```python
from build123d import *

# Parameters (mm, degrees)
SKETCH12_W           = 12.7
SKETCH12_H           = 41.275
SKETCH12_R           = 2.5527
BOSS_EXTRUDE5_DEPTH  = 12.7
SKETCH13_R           = 2.0193
CUT_EXTRUDE3_DEPTH   = 13.7
SKETCH107_W          = 9.525
SKETCH107_H          = 11.1125
SKETCH107_R          = 2.0193
BOSS_EXTRUDE34_DEPTH = 12.7
SKETCH112_R          = 1.651
CUT_EXTRUDE58_DEPTH  = 13.7
FILLET43_R           = 2.54
FILLET44_R           = 0.635


with BuildPart() as part:
    # Sketch12 → Boss-Extrude5 (new body)
    with BuildSketch(Plane(origin=(0, 19.05, 0), x_dir=(1, 0, 0), z_dir=(0, 1, 0))):
        with Locations((-98.425, -57.012186106)):
            Rectangle(SKETCH12_W, SKETCH12_H)
        with Locations((-98.425, -63.362186106)):
            Circle(SKETCH12_R, mode=Mode.SUBTRACT)
        with Locations((-98.425, -50.662186106)):
            Circle(SKETCH12_R, mode=Mode.SUBTRACT)
    extrude(amount=-BOSS_EXTRUDE5_DEPTH)

    # Sketch13 → Cut-Extrude3 (cut, through all)
    with BuildSketch(Plane.ZY.offset(104.775)):
        with Locations((44.312186106, 12.7)):
            Circle(SKETCH13_R)
        with Locations((57.012186106, 12.7)):
            Circle(SKETCH13_R)
        with Locations((69.712186106, 12.7)):
            Circle(SKETCH13_R)
    extrude(amount=-CUT_EXTRUDE3_DEPTH, mode=Mode.SUBTRACT)

    # Sketch107 → Boss-Extrude34 (add, through all)
    with BuildSketch(Plane(origin=(-92.075, 0, 0), x_dir=(0, 0, -1), z_dir=(1, 0, 0))):
        with Locations((-72.887186106, 24.60625)):
            Rectangle(SKETCH107_W, SKETCH107_H)
        with Locations((-72.887186106, 24.60625)):
            Circle(SKETCH107_R, mode=Mode.SUBTRACT)
    extrude(amount=-BOSS_EXTRUDE34_DEPTH)

    # Sketch112 → Cut-Extrude58 (cut, through all)
    with BuildSketch(Plane.ZY.offset(104.775)):
        with Locations((50.662186106, 20.32)):
            Circle(SKETCH112_R)
        with Locations((63.362186106, 20.32)):
            Circle(SKETCH112_R)
    extrude(amount=-CUT_EXTRUDE58_DEPTH, mode=Mode.SUBTRACT)

    # Fillet43
    fillet43_edges = [part.edges().sort_by_distance(p)[0] for p in [
        (-98.425, 19.05, 68.124686106),
    ]]
    fillet(fillet43_edges, radius=FILLET43_R)

    # Fillet44
    fillet44_edges = [part.edges().sort_by_distance(p)[0] for p in [
        (-98.425, 6.35, 36.374686106),
        (-98.425, 30.1625, 77.649686106),
        (-98.425, 30.1625, 68.124686106),
        (-98.425, 6.35, 77.649686106),
        (-98.425, 19.05, 36.374686106),
    ]]
    fillet(fillet44_edges, radius=FILLET44_R)


solid = part.part
```
Model file for the job. Use its own axes, mm. A direction names the side the tool comes from. Coordinates: 2 decimals unless noted, no trailing zeros. Loops run counter-clockwise (first coordinate to the right, second up) from the corner with the lowest first, then second, coordinate; pieces in that order, holes last. Notation, with made-up numbers: (81, -7) - (112, -7) arc R16 ccw to (112, 19) - close; hole circle Ø9 at (79, 34.5). An arc over 180 degrees is marked (long way). Answer as a JSON object with one key per item and string values. Group by question number.
(1) Two-plate mould, pull along Y, no slides. Class faces 3 (the face through (-94.12, 18.67, 63.35)), 4 (the face through (-104.775, 16, 62)), 5 (the face through (-98.336, 24.695, 74.905)), 6 (the face through (-98.514, 12.789, 42.295)): released by +Y, released by -Y, zero draft, split by the parting line, or undercut.
(2) Probe line 1 along Z through (x, y) = (-95, 13.25); line 2 along Y through (x, z) = (-93.25, 43); line 3 along Z through (x, y) = (-102, 12.25). List the from-to ranges inside material, lowest first.
(3) Cut at A-A (y = 12.7). Give the cut face in (x, z) (3 decimals).
(4) Cut at D-D (y = 16.75). Give the cut face in (x, z) (3 decimals), then the cut area to 3 significant figures.
(5) Tool access for faces 1 (the face through (-99, 19.05, 57)), 2 (the face through (-99, 13, 36.375)): list every direction of +Z, -Z, +X, -X, +Y, -Y with a clear straight run to the whole face (end or side of a thin tool).
(6) Flat gauge pins, fed straight in: pin 1 (5.5 mm diameter, centred on x = -99.5, z = 59.5, fed in from +Y); pin 2 (6.5 mm diameter, centred on x = -100.5, y = 23.5, fed in from -Z). Where does each tip first touch, or does it go through?
(7) Cut at C-C (x = -98.25). State how many separate pieces and enclosed holes the cut face has, then the cut area to 3 significant figures.
Geometry says:
{
 "1": {"face 3": "released by +Y", "face 4": "zero draft", "face 5": "undercut", "face 6": "undercut"},
 "2": {"line 1": "z = 36.37 to 42.37, 46.26 to 55.07, 58.96 to 67.77, 71.66 to 77.65", "line 2": "y = 6.35 to 11.17, 14.23 to 19.05", "line 3": "z = 36.37 to 42.34, 46.28 to 55.04, 58.98 to 67.74, 71.68 to 77.65"},
 "3": {"outline": "(-104.775, 36.375) - (-92.075, 36.375) - (-92.075, 42.293) - (-104.775, 42.293) - close; (-104.775, 46.331) - (-92.075, 46.331) - (-92.075, 54.993) - (-104.775, 54.993) - close; (-104.775, 59.031) - (-92.075, 59.031) - (-92.075, 67.693) - (-104.775, 67.693) - close; (-104.775, 71.731) - (-92.075, 71.731) - (-92.075, 77.65) - (-104.775, 77.65) - close; hole circle Ø5.105 at (-98.425, 50.662); hole circle Ø5.105 at (-98.425, 63.362)"},
 "4": {"outline": "(-104.775, 36.375) - (-92.075, 36.375) - (-92.075, 77.65) - (-104.775, 77.65) - close; hole circle Ø5.105 at (-98.425, 50.662); hole circle Ø5.105 at (-98.425, 63.362)", "area": "483 mm^2"},
 "5": {"face 1": "-Z, +X, -X, +Y", "face 2": "-Z, +X, -X, +Y, -Y"},
 "6": {"pin 1": "stops at y = 19.05", "pin 2": "stops at z = 67.74"},
 "7": {"separate pieces": "3", "enclosed holes": "4", "area": "450 mm^2"}
}
